Geometry check sheet. Reference: the model listing, model coordinates, mm. A direction names the side the tool comes from. Coordinates: 2 decimals unless noted, no trailing zeros. Loops run counter-clockwise (first coordinate to the right, second up) from the corner with the lowest first, then second, coordinate; pieces in that order, holes last.
from build123d import *

# Parameters (mm, degrees)
SKIZZE1_W                        = 205
SKIZZE1_H                        = 25
AUFSATZ_LINEAR_AUSTRAGEN1_DEPTH  = 26
SKIZZE2_W                        = 2.5
SKIZZE2_H                        = 25
AUFSATZ_LINEAR_AUSTRAGEN2_DEPTH  = 5
F_18_0_18_DURCHMESSER_BOHRUNG1_D = 18


with BuildPart() as part:
    # Skizze1 → Aufsatz-Linear austragen1 (new body)
    with BuildSketch(Plane.XY):
        with Locations((102.5, 12.5)):
            Rectangle(SKIZZE1_W, SKIZZE1_H)
    extrude(amount=AUFSATZ_LINEAR_AUSTRAGEN1_DEPTH)

    # Skizze2 → Aufsatz-Linear austragen2 (add)
    with BuildSketch(Plane(origin=(0, 0, 0), x_dir=(-1, 0, 0), z_dir=(0, 0, -1))):
        with Locations((-1.25, 12.5)):
            Rectangle(SKIZZE2_W, SKIZZE2_H)
        with Locations((-203.75, 12.5)):
            Rectangle(SKIZZE2_W, SKIZZE2_H)
    extrude(amount=AUFSATZ_LINEAR_AUSTRAGEN2_DEPTH)

    # Ø18.0 (18) Durchmesser Bohrung1 (through all)
    with Locations(Plane(origin=(0, 0, 0), x_dir=(-1, 0, 0), z_dir=(0, 0, -1))):
        with Locations((-32.344324412, 12.5), (-72.588665447, 12.5), (-112.561085259, 12.5), (-152.805426293, 12.5)):
            Hole(F_18_0_18_DURCHMESSER_BOHRUNG1_D / 2)


solid = part.part
1) Section check D-D on x = 19.5. Record the cut outline in (y, z).
Data:
outline: (0, 0) - (25, 0) - (25, 26) - (0, 26) - close
2) Material ranges on probe 1 along X at (y, z) = (11, -2); probe 2 along X at (y, z) = (5, 14.5); probe 3 along X at (y, z) = (20.25, 20.5), recorded low to high.
Data:
probe 1: x = 0 to 2.5, 202.5 to 205
probe 2: x = 0 to 27.37, 37.32 to 67.61, 77.56 to 107.59, 117.54 to 147.83, 157.78 to 205
probe 3: x = 0 to 27.77, 36.92 to 68.01, 77.16 to 107.99, 117.14 to 148.23, 157.38 to 205
3) Section check A-A on y = 12.5. Record the cut outline in (x, z), and give its area (3 significant figures).
Data:
outline: (0, -5) - (2.5, -5) - (2.5, 0) - (23.34, 0) - (23.34, 26) - (0, 26) - close; (41.34, 0) - (63.59, 0) - (63.59, 26) - (41.34, 26) - close; (81.59, 0) - (103.56, 0) - (103.56, 26) - (81.59, 26) - close; (121.56, 0) - (143.81, 0) - (143.81, 26) - (121.56, 26) - close; (161.81, 0) - (202.5, 0) - (202.5, -5) - (205, -5) - (205, 26) - (161.81, 26) - close
area: 3,480 mm2
4) Section check B-B on z = 9.5. Record the cut outline in (x, y), and give its area (3 significant figures).
Data:
outline: (0, 0) - (205, 0) - (205, 25) - (0, 25) - close; hole circle Ø18 at (32.34, 12.5); hole circle Ø18 at (72.59, 12.5); hole circle Ø18 at (112.56, 12.5); hole circle Ø18 at (152.81, 12.5)
area: 4,110 mm2
5) Section check C-C on x = 108.5. Record the cut outline in (y, z), and give its area (3 significant figures).
Data:
outline: (0, 0) - (4.47, 0) - (4.47, 26) - (0, 26) - close; (20.53, 0) - (25, 0) - (25, 26) - (20.53, 26) - close
area: 232 mm2
6) Access from +Z, -Z, +X, -X, +Y, -Y to the whole of each face (thin tool, end or side, straight path). Record for faces 4 (the flat face through (2.5, 12, -2)), 5 (the flat face through (101, 13, 26)).
Data:
face 4: -Z, +Y, -Y
face 5: +Z, +X, -X, +Y, -Y
7) Mould release check, pull along Y, two halves, no side actions. Record for faces 1 (the flat face through (104, 0, 11)), 2 (the flat face through (101, 13, 0)), 3 (the cylindrical face through (103.57, 12.9, 13.18)): +Y half, -Y half, draft (parallel to the pull), parting line (faces both ways), or undercut.
Data:
face 1: -Y half
face 2: draft
face 3: undercut
